Study the drawing (mm; zero at the part's minimum x, y, z) and answer. Give positions to 0.01 mm unless a question says otherwise; leave off trailing zeros. Write each loop counter-clockwise with the first axis right and the second up, starting at its lowest first coordinate (ties: lowest second). Pieces come first, ordered by that corner, then holes. Notation, with made-up numbers: (-15, 1.5) - (23, 1.5) arc R14 ccw to (23, 28.5) - close; hole circle Ø11 at (15.25, 24). An arc over 180 degrees is marked (long way). Return JSON: item names as keys, results as strings.
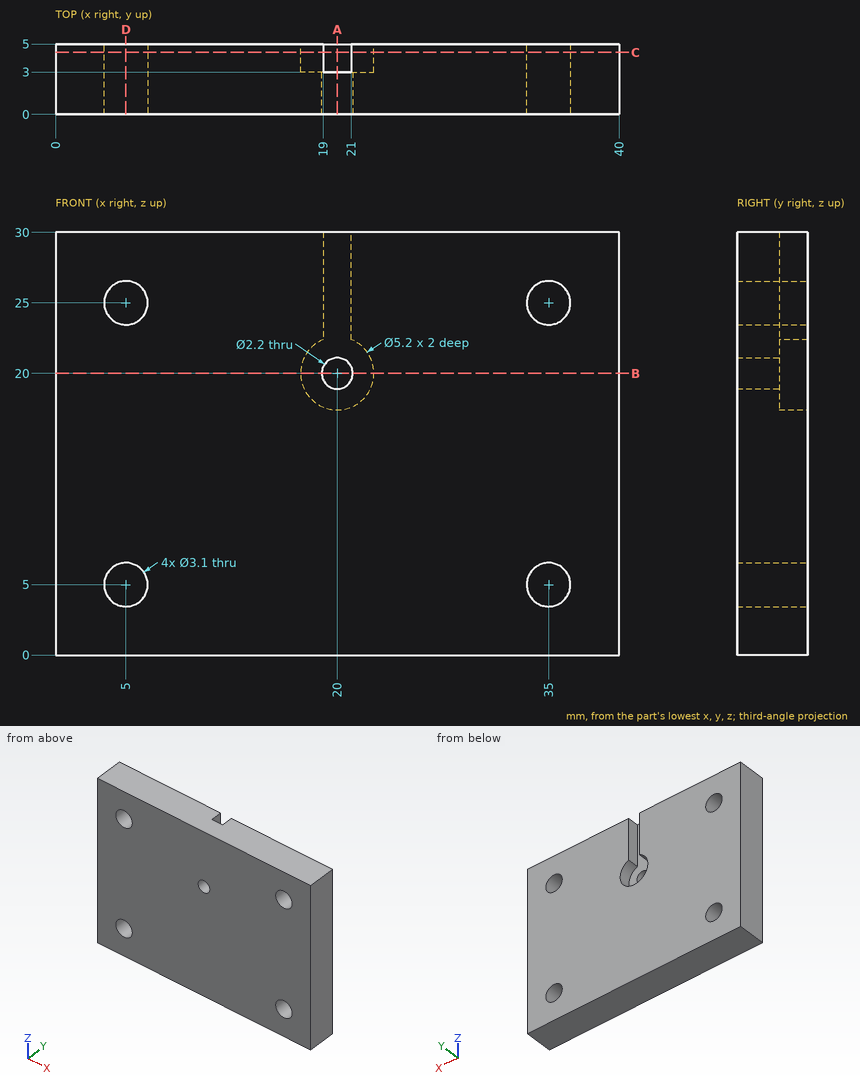
Item 1: A cutting plane is placed at A-A on x = 20. Determine the outline of the cut face in (y, z), then the cut area to 3 significant figures.
Answer below:
{"outline": "(0, 0) - (5, 0) - (5, 17.4) - (3, 17.4) - (3, 18.9) - (0, 18.9) - close; (0, 21.1) - (3, 21.1) - (3, 30) - (0, 30) - close", "area": "118 mm²"}
Item 2: A cutting plane is placed at C-C on y = 4.4. Determine the outline of the cut face in (x, z), then the cut area to 3 significant figures.
Answer below:
{"outline": "(0, 0) - (40, 0) - (40, 30) - (21, 30) - (21, 22.4) arc R2.6 cw (long way) to (19, 22.4) - (19, 30) - (0, 30) - close; hole circle Ø3.1 at (5, 5); hole circle Ø3.1 at (5, 25); hole circle Ø3.1 at (35, 5); hole circle Ø3.1 at (35, 25)", "area": "1,130 mm²"}
Item 3: A cutting plane is placed at B-B on z = 20. Determine the outline of the cut face in (x, y), then the cut area to 3 significant figures.
Answer below:
{"outline": "(0, 0) - (18.9, 0) - (18.9, 3) - (17.4, 3) - (17.4, 5) - (0, 5) - close; (21.1, 0) - (40, 0) - (40, 5) - (22.6, 5) - (22.6, 3) - (21.1, 3) - close", "area": "183 mm²"}
Item 4: Consider L1, parallel to Z at x = 35, y = 1.2; L2, parallel to X at y = 4.1, z = 20; L3, parallel to Z at x = 20, y = 2.1. Determine where each line is inside the solid, lowest interval first.
Answer below:
{"L1": "z = 0 to 3.45, 6.55 to 23.45, 26.55 to 30", "L2": "x = 0 to 17.4, 22.6 to 40", "L3": "z = 0 to 18.9, 21.1 to 30"}
Item 5: Flat-ended cylindrical pins translate along their axes: P1, Ø2.5, axis at x = 5, z = 5, coming from the +Y side; P2, Ø1, axis at y = 4, z = 25, coming from the -X side; P3, Ø2.5, axis at x = 20, z = 20, coming from the +Y side. Find the tip coordinate at first contact, or state that the pin passes through.
Answer below:
{"P1": "passes through", "P2": "stops at x = 0", "P3": "stops at y = 3"}
Item 6: A cutting plane is placed at D-D on x = 5. Determine the outline of the cut face in (y, z).
Answer below:
{"outline": "(0, 0) - (5, 0) - (5, 3.45) - (0, 3.45) - close; (0, 6.55) - (5, 6.55) - (5, 23.45) - (0, 23.45) - close; (0, 26.55) - (5, 26.55) - (5, 30) - (0, 30) - close"}
